Geometry check sheet. Reference: drawing and pictorial views, mm from the part's lowest x, y, z. A direction names the side the tool comes from. Give positions to 0.01 mm unless a question says otherwise; leave off trailing zeros. Loops run counter-clockwise (first coordinate to the right, second up) from the corner with the lowest first, then second, coordinate; pieces in that order, holes last. Notation, with made-up numbers: (-10.5, -15) -> (8.5, -15) arc R35 cw to (8.5, 18) -> close; hole circle Ø8 at (71, 51.25). An arc over 180 degrees is marked (long way). Answer in a Markdown table with one row per item. Add a question column.
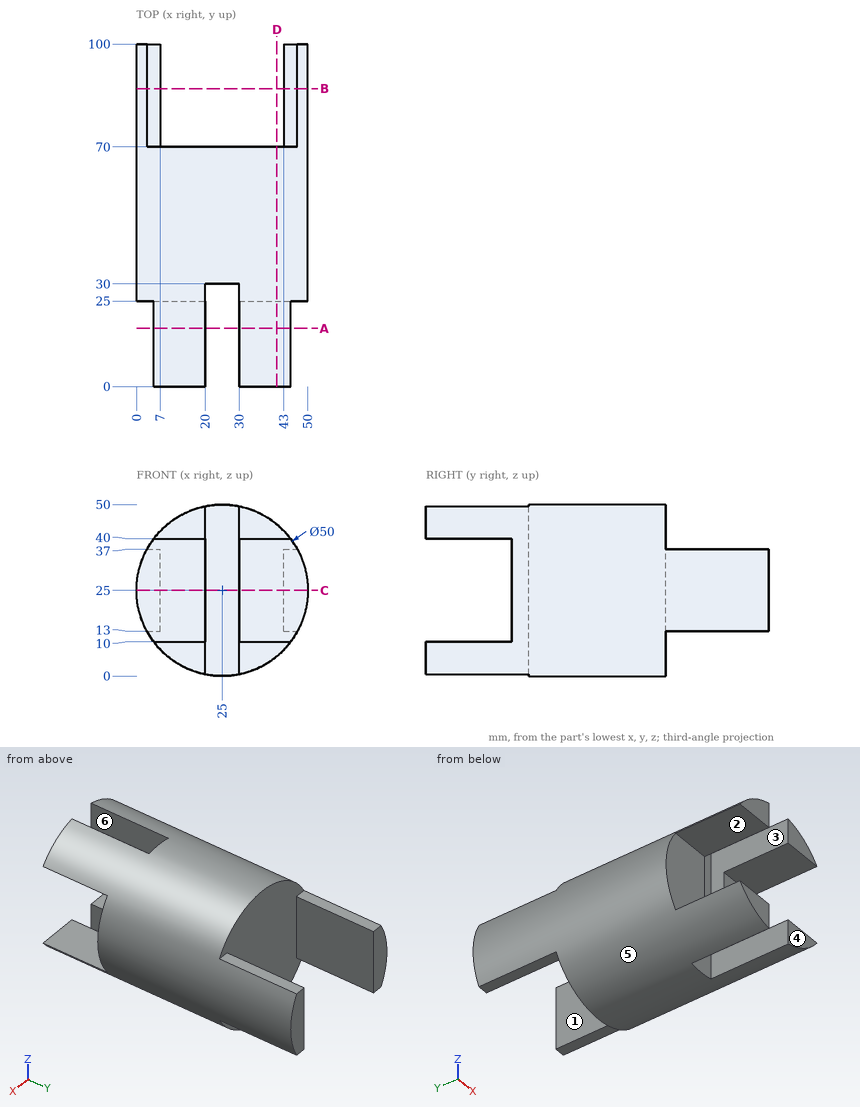
1. Gauge pin test, flat ends, axial feed: pin 1 Ø1 at (x, z) = (16, 45) entering from +Y; pin 2 Ø2 at (x, y) = (32, 47.5) entering from +Z; pin 3 Ø1 at (x, z) = (40, 17) entering from -Y. Record the tip position at first contact, or that the pin passes through.
2. Sectioned sample at D-D (x = 41). Enter the section's corners in (y, z), plus the area to 3 significant figures.
3. Sectioned sample at B-B (y = 87). Enter the section's corners in (x, z).
4. Release check for a two-part mould opening along X. For the marked faces 4, 5 and 6 record: released by +X, released by -X, zero draft, split by the parting line, or undercut.
5. Access from +Z, -Z, +X, -X, +Y, -Y to the whole of each face (thin tool, end or side, straight path). Record for the marked faces 1, 2 and 3.
6. Sectioned sample at C-C (z = 25). Enter the section's corners in (x, y), plus the area to 3 significant figures.
7. Material ranges on L1, parallel to Y at x = 13, z = 35.5; L2, parallel to Z at x = 40.5, y = 17.5; L3, parallel to X at y = 79.5, z = 14, recorded low to high. Write a range as from..to.
8. Sectioned sample at A-A (y = 17). Enter the section's corners in (x, z).
Response:
| question | item | result |
|---|---|---|
| 1 | pin 1 | stops at y = 70 |
| 1 | pin 2 | stops at z = 49.27 |
| 1 | pin 3 | stops at y = 25 |
| 2 | outline | (0, 5.79) -> (70, 5.79) -> (70, 44.21) -> (0, 44.21) -> (0, 40) -> (25, 40) -> (25, 10) -> (0, 10) -> close |
| 2 | area | 1,940 mm2 |
| 3 | outline | (3.07, 13) -> (7, 13) -> (7, 37) -> (3.07, 37) arc R25 ccw to start; (43, 13) -> (46.93, 13) arc R25 ccw to (46.93, 37) -> (43, 37) -> close |
| 4 | face 4 | zero draft |
| 4 | face 5 | split by the parting line |
| 4 | face 6 | undercut |
| 5 | face 1 | +Z, -Z, +Y |
| 5 | face 2 | +X, -X, -Y |
| 5 | face 3 | +Z, -Z, -Y |
| 6 | outline | (0, 25) -> (20, 25) -> (20, 30) -> (30, 30) -> (30, 25) -> (50, 25) -> (50, 100) -> (43, 100) -> (43, 70) -> (7, 70) -> (7, 100) -> (0, 100) -> close |
| 6 | area | 2,620 mm2 |
| 7 | L1 | y = 25..70 |
| 7 | L2 | z = 5.38..10, 40..44.62 |
| 7 | L3 | x = 2.55..7, 43..47.45 |
| 8 | outline | (5, 10) arc R25 ccw to (20, 0.51) -> (20, 10) -> close; (5, 40) -> (20, 40) -> (20, 49.49) arc R25 ccw to start; (30, 0.51) arc R25 ccw to (45, 10) -> (30, 10) -> close; (30, 40) -> (45, 40) arc R25 ccw to (30, 49.49) -> close |
